Study the drawing (mm; zero at the part's minimum x, y, z) and answer. A direction names the side the tool comes from. Coordinates: 2 decimals unless noted, no trailing zeros. Write each loop counter-clockwise with the first axis right and the second up, starting at its lowest first coordinate (ties: lowest second). Pieces come first, ordered by that corner, then holes. Notation, with made-up numbers: (65.5, 62) -> (118.5, 62) arc R25 cw to (118.5, 93) -> close; hole circle Ø3 at (19.5, -14.5). An arc over 180 degrees is marked (long way). Write item = value, one per line. Start each with the question number.
1) Find the intervals of material crossed by line 1 along Y through (x, z) = (37.5, 21.5); line 2 along X through (y, z) = (21, 66); line 3 along Z through (x, y) = (34, 9.5), in increasing order. Write a range as from..to.
2) Section C-C (z = 52.5) is taken. Determine the outline of the cut face in (x, y).
3) A tool of negligible diameter and unlimited length cuts with its end or side. For the marked faces 1 and 2, from which of +Z, -Z, +X, -X, +Y, -Y can it reach the whole face along a straight path? Write none if from no direction.
4) Section A-A (y = 21.5) is taken. Determine the outline of the cut face in (x, z), plus the area to 3 significant figures.
5) Section B-B (x = 37) is taken. Determine the outline of the cut face in (y, z).
6) Section D-D (x = 21.5) is taken. Determine the outline of the cut face in (y, z), plus the area to 3 significant figures.
7) Flat-ended cylindrical pins translate along their axes: pin 1 Ø8 at (x, y) = (32.5, 29) entering from -Z; pin 2 Ø1 at (x, z) = (37.5, 41.5) entering from +Y; pin 3 Ø4 at (y, z) = (35.5, 59) entering from +X; pin 4 Ø5 at (x, z) = (24.5, 26.5) entering from +Y. Find the tip coordinate at first contact, or state that the pin passes through.
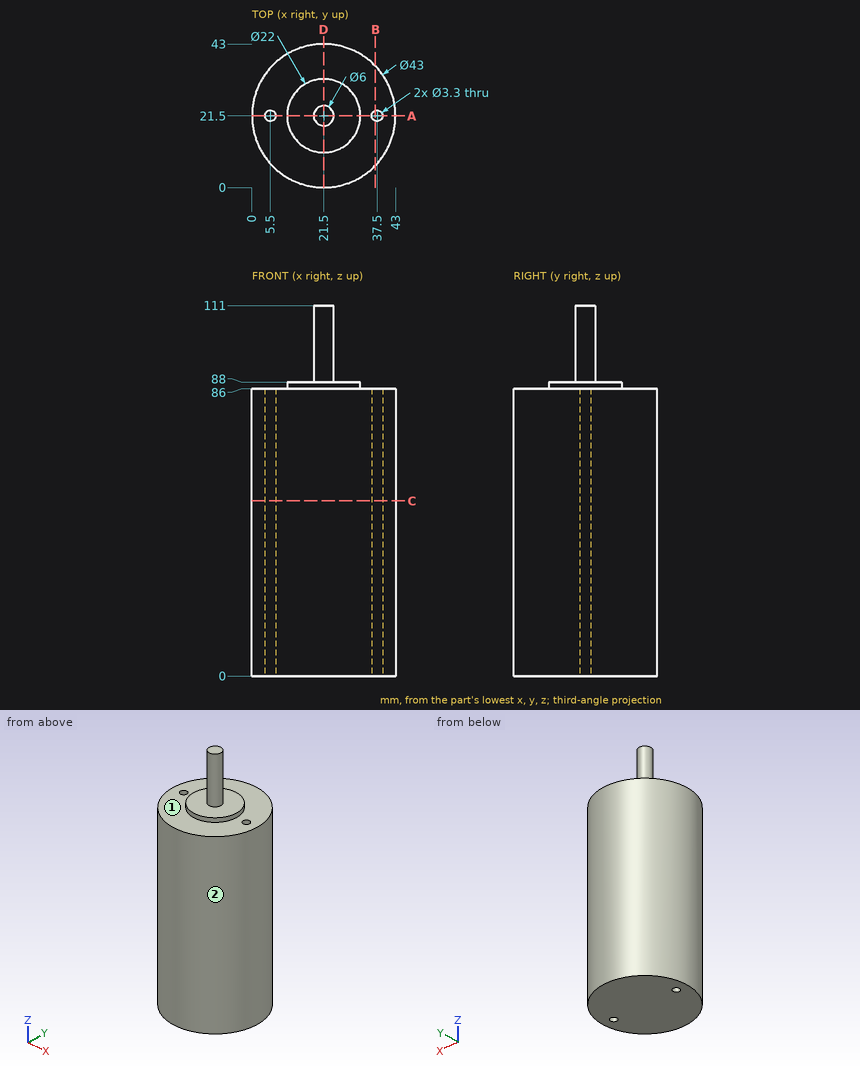
Answer key:
q1.line_1 = 7.14..19.85, 23.15..35.86
q1.line_2 = 0.01..3.93, 7.07..35.93, 39.07..42.99
q1.line_3 = 0..86
q2.outline = circle Ø43 at (21.5, 21.5); hole circle Ø3.3 at (5.5, 21.5); hole circle Ø3.3 at (37.5, 21.5)
q3.face_1 = +Z
q3.face_2 = +Z, -Z
q4.outline = (0, 0) -> (3.85, 0) -> (3.85, 86) -> (0, 86) -> close; (7.15, 0) -> (35.85, 0) -> (35.85, 86) -> (32.5, 86) -> (32.5, 88) -> (24.5, 88) -> (24.5, 111) -> (18.5, 111) -> (18.5, 88) -> (10.5, 88) -> (10.5, 86) -> (7.15, 86) -> close; (39.15, 0) -> (43, 0) -> (43, 86) -> (39.15, 86) -> close
q4.area = 3,310 mm^2
q5.outline = (6.6, 0) -> (19.93, 0) -> (19.93, 86) -> (6.6, 86) -> close; (23.07, 0) -> (36.4, 0) -> (36.4, 86) -> (23.07, 86) -> close
q6.outline = (0, 0) -> (43, 0) -> (43, 86) -> (32.5, 86) -> (32.5, 88) -> (24.5, 88) -> (24.5, 111) -> (18.5, 111) -> (18.5, 88) -> (10.5, 88) -> (10.5, 86) -> (0, 86) -> close
q6.area = 3,880 mm^2
q7.pin_1 = 0
q7.pin_2 = 36.4
q7.pin_3 = 39.34
q7.pin_4 = 42.99
